from build123d import *

# Parameters (mm, degrees)
SKETCH_1_R      = 1.5
SKETCH_1_R_2    = 1
SKETCH_1_W      = 3.04
SKETCH_1_H      = 8.04
EXTRUDE_1_DEPTH = 3


with BuildPart() as part:
    # 草图1 → 凸台-拉伸1 (new body)
    with BuildSketch(Plane.XY):
        with BuildLine():
            Line((56, -336.18), (56, -441))
            ThreePointArc((56, -441), (56.535533906, -448.535533906), (49, -448))
            Line((49, -448), (4, -448))
            ThreePointArc((4, -448), (-3.535533906, -448.535533906), (-3, -441))
            Line((-3, -441), (-3, -438.832903769))
            Line((-3, -438.832903769), (-3, -429.017949192))
            Line((-3, -429.017949192), (-3, -336.18))
            ThreePointArc((-3, -336.18), (-5, -332.18), (-3, -328.18))
            Line((-3, -328.18), (-3, -116.82))
            ThreePointArc((-3, -116.82), (-5, -112.82), (-3, -108.82))
            Line((-3, -108.82), (-3, -4))
            ThreePointArc((-3, -4), (-5, 0), (-3, 4))
            Line((-3, 4), (-3, 51))
            ThreePointArc((-3, 51), (-4, 58), (3, 59))
            Line((3, 59), (56.535533906, 3.535533906))
            ThreePointArc((56.535533906, 3.535533906), (57.987421044, -0.3544451), (56, -4))
            Line((56, -4), (56, -328.18))
            ThreePointArc((56, -328.18), (58, -332.18), (56, -336.18))
        make_face()
        Circle(SKETCH_1_R, mode=Mode.SUBTRACT)
        with Locations((0, -445)):
            Circle(SKETCH_1_R, mode=Mode.SUBTRACT)
        with Locations((0, -332.18)):
            Circle(SKETCH_1_R, mode=Mode.SUBTRACT)
        with Locations(Location((53, -332.18, 0), (0, 0, 180))):
            Circle(SKETCH_1_R, mode=Mode.SUBTRACT)
        with Locations(Location((53, -445, 0), (0, 0, 180))):
            Circle(SKETCH_1_R, mode=Mode.SUBTRACT)
        with Locations(Location((53, 0, 0), (0, 0, 180))):
            Circle(SKETCH_1_R, mode=Mode.SUBTRACT)
        with Locations((5, -399.337663182)):
            Circle(SKETCH_1_R_2, mode=Mode.SUBTRACT)
        with Locations((0, 55)):
            Circle(SKETCH_1_R, mode=Mode.SUBTRACT)
        with Locations((0, -112.82)):
            Circle(SKETCH_1_R, mode=Mode.SUBTRACT)
        with BuildLine():
            Line((6.938150971, 3), (41.969807465, 3))
            ThreePointArc((41.969807465, 3), (44.729078046, 4.822534134), (44.135772081, 8.07571609))
            Line((44.135772081, 8.07571609), (8.325634331, 45.44281635))
            ThreePointArc((8.325634331, 45.44281635), (5.012233456, 46.138993121), (3.160320545, 43.30461382))
            Line((3.160320545, 43.30461382), (3.938801801, 5.937513559))
            ThreePointArc((3.938801801, 5.937513559), (4.839039174, 3.85670122), (6.938150971, 3))
        make_face(mode=Mode.SUBTRACT)
        with BuildLine():
            Line((48, -86.226063366), (48, -438))
            ThreePointArc((48, -438), (47.414213562, -439.414213562), (46, -440))
            Line((46, -440), (11.226944195, -440))
            ThreePointArc((11.226944195, -440), (9.744803089, -439.342854326), (9.236644598, -437.803257741))
            Line((9.236644598, -437.803257741), (44.009700404, -86.029321107))
            ThreePointArc((44.009700404, -86.029321107), (46.098490627, -84.228489939), (48, -86.226063366))
        make_face(mode=Mode.SUBTRACT)
        with BuildLine():
            Line((43.763355402, -7.196742259), (8.990299596, -358.970678893))
            ThreePointArc((8.990299596, -358.970678893), (6.901509373, -360.771510061), (5, -358.773936634))
            Line((5, -358.773936634), (5, -7))
            ThreePointArc((5, -7), (5.585786438, -5.585786438), (7, -5))
            Line((7, -5), (41.773055805, -5))
            ThreePointArc((41.773055805, -5), (43.255196911, -5.657145674), (43.763355402, -7.196742259))
        make_face(mode=Mode.SUBTRACT)
        with Locations((53, -56.41)):
            Rectangle(SKETCH_1_W, SKETCH_1_H, mode=Mode.SUBTRACT)
        with Locations((0, -56.41)):
            Rectangle(SKETCH_1_W, SKETCH_1_H, mode=Mode.SUBTRACT)
        with Locations((53, -278.91)):
            Rectangle(SKETCH_1_W, SKETCH_1_H, mode=Mode.SUBTRACT)
        with Locations((0, -278.91)):
            Rectangle(SKETCH_1_W, SKETCH_1_H, mode=Mode.SUBTRACT)
    extrude(amount=EXTRUDE_1_DEPTH)


solid = part.part
Geometry: final body of the model. Coordinates: model frame, mm. A direction names the side the tool comes from. Round coordinates to 2 decimals unless told otherwise and drop trailing zeros. Order: outer loops, then holes, each group sorted by start corner. A loop starts at its lowest first (then second) coordinate and runs counter-clockwise, first axis right, second up.
Q1. Material intervals for probe 1 along X at (y, z) = (-445, 2.25); probe 2 along X at (y, z) = (-144, 2.75); probe 3 along Y at (x, z) = (53, 1.4), sorted ascending.
Result sheet:
probe 1: x = -5 to -1.5, 1.5 to 51.5, 54.5 to 58
probe 2: x = -3 to 5, 30.24 to 38.28, 48 to 56
probe 3: y = -450 to -446.5, -443.5 to -333.68, -330.68 to -282.93, -274.89 to -60.43, -52.39 to -1.5, 1.5 to 7.2
Q2. Section B-B, the plane x = 22. Output: boundary loops of the cut face in (y, z), and give its area (3 significant figures).
Result sheet:
outline: (-448, 0) - (-440, 0) - (-440, 3) - (-448, 3) - close; (-308.69, 0) - (-227.36, 0) - (-227.36, 3) - (-308.69, 3) - close; (-5, 0) - (3, 0) - (3, 3) - (-5, 3) - close; (31.17, 0) - (39.32, 0) - (39.32, 3) - (31.17, 3) - close
area: 316 mm2
Q3. Access query for faces 1 (the face through (29, -175, 0)), 2 (the face through (26.62, -180.62, 1.48)). Directions: +Z, -Z, +X, -X, +Y, -Y. A direction counts if a zero-diameter tool reaches every point of the face in a straight line with its end or side. Return the directions, or none.
Result sheet:
face 1: -Z, +X, -X, +Y, -Y
face 2: +Z, -Z
Q4. Section C-C, the plane z = 1.75. Give the number of separate pieces and of enclosed holes in the cut face, and give its area (3 significant figures).
Result sheet:
separate pieces: 1
enclosed holes: 16
area: 12,100 mm2
Q5. Section A-A, the plane y = -154. Output: boundary loops of the cut face in (x, z), and give its area (3 significant figures).
Result sheet:
outline: (-3, 0) - (5, 0) - (5, 3) - (-3, 3) - close; (29.25, 0) - (37.29, 0) - (37.29, 3) - (29.25, 3) - close; (48, 0) - (56, 0) - (56, 3) - (48, 3) - close
area: 72.1 mm2
Q6. Mould query, pull axis X, two halves, no side actions, for faces 3 (the face through (-4, 58, 1)), 4 (the face through (57, -448, 1)), 5 (the face through (29, -175, 3)). Classes: released by +X, released by -X, zero draft, split by the parting line, or undercut.
Result sheet:
face 3: split by the parting line
face 4: undercut
face 5: zero draft
Q7. Pin query (flat end, axial travel): pin 1 (0.9 mm diameter, centred on y = -55, z = 1.5, fed in from +X); pin 2 (1.5 mm diameter, centred on y = -349.5, z = 2, fed in from -X); pin 3 (1.5 mm diameter, centred on x = 8.5, z = 0.5, fed in from +Y). Return the tip coordinate at first contact, or that it passes through.
Result sheet:
pin 1: stops at x = 56
pin 2: stops at x = -3
pin 3: stops at y = 54.08
